Read the model definition and answer for the solid it produces. Units are mm, in the model's axes. Face numbers are marked on the shaded views. A direction names the side the tool comes from. Coordinates: 2 decimals unless noted, no trailing zeros. Order: outer loops, then holes, each group sorted by start corner. A loop starts at its lowest first (then second) coordinate and runs counter-clockwise, first axis right, second up. Notation, with made-up numbers: M -16,-25.75 L -2,-25.75 A32 ccw -2,13.25 Z; hole C -32,2.25 d2. An arc over 180 degrees is marked long. One line per question, with ' | ' between items. Start each with the question number.
1) Find section B-B, the plane y = 10.5. Write down the section's boundary in (x, z).
2) Find section D-D, the plane x = 4. Write down the section's boundary in (y, z), plus the area to 3 significant figures.
3) Find section C-C, the plane y = 23.5. Write down the section's boundary in (x, z).
4) Find section A-A, the plane x = 30. Write down the section's boundary in (y, z), plus the area to 3 significant figures.
5) A tool of negligible diameter and unlimited length cuts with its end or side. For the marked faces 4 and 5, from which of +Z, -Z, +X, -X, +Y, -Y can it reach the whole face along a straight path? Write none if from no direction.
6) Consider probe 1 along X at (y, z) = (50.25, 10); probe 2 along Z at (x, y) = (16, 58.5); probe 3 along X at (y, z) = (5, 10). Determine where each line is inside the solid, lowest interval first.
7) Given P1, Ø3, axis at x = 27.5, y = 48.5, coming from the -Z side; P2, Ø1.2, axis at x = 16.5, z = 11, coming from the +Y side; P3, Ø3, axis at x = 37, z = 17, coming from the -Y side; P4, Ø8, axis at y = 9, z = 8, coming from the +X side, each flat-ended and moving along its own axis, determine where each tip first touches the part or whether it passes through.
8) The mould has two halves that part along Y. Classify the marked faces 1, 2 and 3: +Y half, -Y half, draft (parallel to the pull), parting line (faces both ways), or undercut.
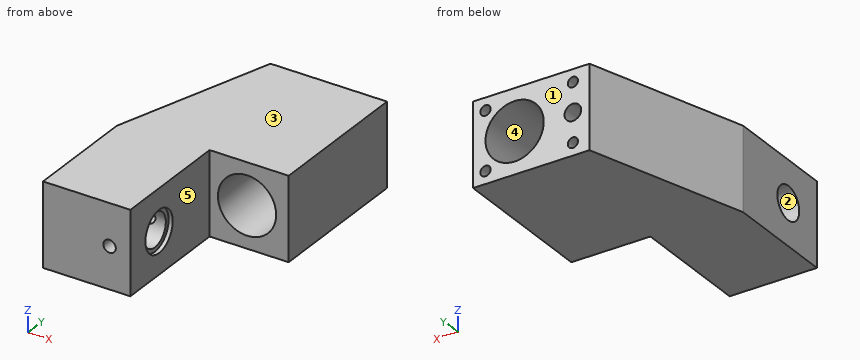
Autodesk Inventor part; units mm, degrees
ref_plane "Arbeitsebene1" through (0, 12, 0) normal (0, 1, 0) x (-1, 0, 0)
ref_plane "Arbeitsebene2" through (26.5, 0, 0) normal (1, 0, 0) x (0, 1, 0)
ref_plane "XY Plane" through (0, 0, 0) normal (0, 0, 1) x (1, 0, 0)
sketch "Skizze1" plane through (0, 0, 0) normal (0, 0, 1) x (1, 0, 0)
  line L0 (0, 0) -> (0, 27)
  line L1 (0, 27) -> (12, 65)
  line L2 (12, 65) -> (40, 65)
  line L3 (40, 65) -> (40, 29)
  line L4 (40, 29) -> (21, 29)
  line L5 (21, 29) -> (21, 0)
  line L6 (21, 0) -> (0, 0)
  dimension "d0" = 65
  dimension "d1" = 21
  dimension "d2" = 29
  dimension "d3" = 38
  dimension "d4" = 28
  dimension "d5" = 12
extrude "Extrusion1" add sketch "Skizze1" along normal blind 20
sketch "Skizze3" plane through (12, 65, 0) normal (0, 1, 0) x (1, 0, 0)
  line L0 (0, 0) -> (0, -20)
  line L1 (28, 0) -> (28, -20)
  point P0 (-12, 0)
  point P1 (18, -10)
  point P2 (28, -10)
  dimension "d16" = 10
hole "Bohrung2" at (30, 65, 10) direction (0, -1, 0) diameter 14 end through all
sketch "Skizze4" plane through (12, 65, 0) normal (0, 1, 0) x (1, 0, 0)
  line L0 (0, 0) -> (0, -20)
  line L1 (28, 0) -> (28, -20)
  point P0 (-12, 0)
  point P1 (4, -10)
  point P2 (28, -10)
  dimension "d24" = 4
hole "Bohrung3" at (16, 65, 10) direction (0, -1, 0) diameter 3 depth 65 counterbore diameter 4 counterbore depth 30
sketch "Skizze5" plane through (21, 0, 0) normal (1, 0, 0) x (0, 0, -1)
  line L0 (0, 0) -> (-20, 0)
  point P0 (-10, 10.5)
  point P1 (-10, 0)
  dimension "d32" = 10.5
hole "Bohrung4" at (21, 10.5, 10) direction (-1, 0, 0) diameter 8 depth 21 counterbore diameter 10 counterbore depth 1
ref_plane "Arbeitsebene1" through (0, 12, 0) normal (0, 1, 0) x (-1, 0, 0)
sketch "Skizze8" plane through (12, 65, 0) normal (0, 1, 0) x (1, 0, 0)
  circle A0 centre (4, -10) radius 2
  circle A1 centre (18, -10) radius 7
  line L0 (28, 0) -> (0, 0)
  line L1 (0, 0) -> (0, -20)
  line L2 (28, -20) -> (0, -20)
  line L3 (28, 0) -> (28, -20)
  line L4 (4, -10) -> (4, -3) construction
  line L5 (4, -10) -> (4, -17) construction
  line L6 (18, -10) -> (9, -10) construction
  line L7 (9, 0) -> (9, -20)
  point P0 (-12, 0)
  dimension "d57" = 14
hole "Bohrung7" at (16, 65, 17) at (16, 65, 3) direction (0, -1, 0) diameter 2.459 depth 9 tip angle 118
ref_plane "Arbeitsebene2" through (26.5, 0, 0) normal (1, 0, 0) x (0, 1, 0)
mirror "Spiegeln2" about plane through (26.5, 0, 0) normal (1, 0, 0) of "Bohrung7"
properties part number "MotorBlock" material "Stahl, galvanisiert"
Report:
1) outline: M 0,0 L 21,0 L 21,5 L 20,5 L 20,6 L 0,6 Z; M 0,14 L 20,14 L 20,15 L 21,15 L 21,20 L 0,20 Z
2) outline: M 0,0 L 39.67,0 L 39.67,20 L 0,20 Z; hole C 10.5,10 d8 | area: 743 mm^2
3) outline: M 0,0 L 21,0 L 21,20 L 0,20 Z; hole C 16,10 d3
4) outline: M 29,0 L 65,0 L 65,3 L 29,3 Z; M 29,17 L 65,17 L 65,20 L 29,20 Z | area: 216 mm^2
5) face 4: +Y, -Y | face 5: +Z, -Z, +X, -Y
6) probe 1: x = 7.34 to 14, 18 to 23, 37 to 40 | probe 2: z = 0 to 1.77, 4.23 to 8, 12 to 15.77, 18.23 to 20 | probe 3: x = 0 to 14.5, 17.5 to 21
7) P1: stops at z = 0 | P2: stops at y = 35 | P3: stops at y = 29 | P4: stops at x = 21
8) face 1: +Y half | face 2: undercut | face 3: draft
